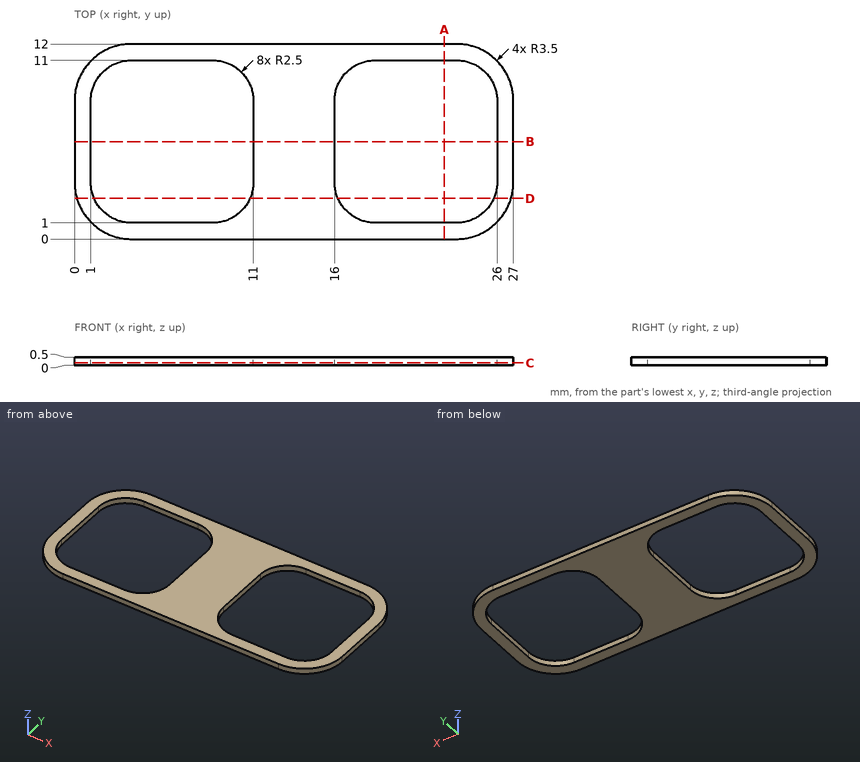
Source: three-view drawing plus pictorial views. Frame: mm from the lowest corner of the part. Round coordinates to 2 decimals unless told otherwise and drop trailing zeros. Loops run counter-clockwise (first coordinate to the right, second up) from the corner with the lowest first, then second, coordinate; pieces in that order, holes last.
Q1. Section A-A on x = 22.75. Return loops of the section in (y, z), plus the area to 3 significant figures.
Q2. Section B-B on y = 6. Return loops of the section in (x, z), plus the area to 3 significant figures.
Q3. Section D-D on y = 2.5. Return loops of the section in (x, z), plus the area to 3 significant figures.
Q4. Section C-C on z = 0.15. Return loops of the section in (x, y).
Q5. Material intervals for L1, parallel to X at y = 4, z = 0.3; L2, parallel to Y at x = 21.75, z = 0.45; L3, parallel to X at y = 2.25, z = 0.3, sorted ascending.
Evaluation:
1. outline: (0, 0) - (1, 0) - (1, 0.5) - (0, 0.5) - close; (11, 0) - (12, 0) - (12, 0.5) - (11, 0.5) - close
1. area: 1.00 mm2
2. outline: (0, 0) - (1, 0) - (1, 0.5) - (0, 0.5) - close; (11, 0) - (16, 0) - (16, 0.5) - (11, 0.5) - close; (26, 0) - (27, 0) - (27, 0.5) - (26, 0.5) - close
2. area: 3.50 mm2
3. outline: (0.15, 0) - (1.21, 0) - (1.21, 0.5) - (0.15, 0.5) - close; (10.79, 0) - (16.21, 0) - (16.21, 0.5) - (10.79, 0.5) - close; (25.79, 0) - (26.85, 0) - (26.85, 0.5) - (25.79, 0.5) - close
3. area: 3.77 mm2
4. outline: (0, 3.5) arc R3.5 ccw to (3.5, 0) - (23.5, 0) arc R3.5 ccw to (27, 3.5) - (27, 8.5) arc R3.5 ccw to (23.5, 12) - (3.5, 12) arc R3.5 ccw to (0, 8.5) - close; hole (1, 3.5) arc R2.5 ccw to (3.5, 1) - (8.5, 1) arc R2.5 ccw to (11, 3.5) - (11, 8.5) arc R2.5 ccw to (8.5, 11) - (3.5, 11) arc R2.5 ccw to (1, 8.5) - close; hole (16, 3.5) arc R2.5 ccw to (18.5, 1) - (23.5, 1) arc R2.5 ccw to (26, 3.5) - (26, 8.5) arc R2.5 ccw to (23.5, 11) - (18.5, 11) arc R2.5 ccw to (16, 8.5) - close
5. L1: x = 0 to 1, 11 to 16, 26 to 27
5. L2: y = 0 to 1, 11 to 12
5. L3: x = 0.23 to 1.33, 10.67 to 16.33, 25.67 to 26.77
